Verification items for the finished model (mm, model axes). Face numbers are marked on the shaded views. A direction names the side the tool comes from. Give positions to 0.01 mm unless a question says otherwise; leave off trailing zeros. Write each loop counter-clockwise with the first axis right and the second up, starting at its lowest first coordinate (ties: lowest second). Pieces come first, ordered by that corner, then holes. Notation, with made-up numbers: (85.5, 9) -> (126.5, 9) arc R26 cw to (126.5, 35) -> close; hole circle Ø3 at (12, -29.75). An arc over 180 degrees is marked (long way). Answer as CSV lines item,"result". Start each with the question number.
1) Sectioned sample at A-A on y = 0. Record the cut outline in (x, z), and give its area (3 significant figures).
2) Sectioned sample at C-C on z = 18.5. Record the cut outline in (x, y), and give its area (3 significant figures).
3) Material ranges on L1, parallel to Y at x = 0, z = 5.3; L2, parallel to Y at x = 0, z = 1.45; L3, parallel to X at y = -5, z = 5.5, recorded low to high.
4) Sectioned sample at D-D on z = 1.75. Record the cut outline in (x, y), and give its area (3 significant figures).
5) Mould release check, pull along Y, two halves, no side actions. Record for the marked faces 4, 5 and 6: released by +Y, released by -Y, zero draft, split by the parting line, or undercut.
6) Tool access check on the marked faces 1, 2 and 3. Record the directions out of +Z, -Z, +X, -X, +Y, -Y that give a thin tool (end or side, any length) a straight path to the whole face; none if there is none.
7) Sectioned sample at B-B on x = 0. Record the cut outline in (y, z).
8) Gauge pin test, flat ends, axial feed: pin 1 Ø3 at (y, z) = (7, 3.5) entering from +X; pin 2 Ø1 at (x, z) = (-1, 15) entering from -Y; pin 3 Ø7.5 at (x, y) = (0, 0) entering from -Z; pin 4 Ø1 at (x, y) = (-5, 4) entering from +Z. Record the tip position at first contact, or that the pin passes through.
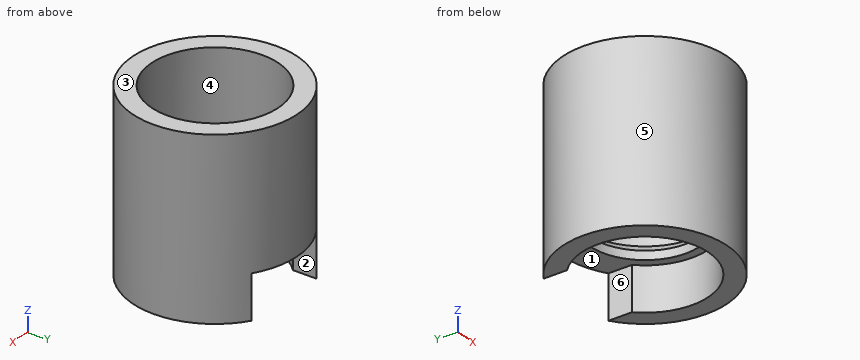
```python
from build123d import *

# Parameters (mm, degrees)
F3_DEPTH = 25


with BuildPart() as f1:
    # F0 (on Front) → F1 (revolve)
    with BuildSketch(Plane.XZ):
        Polygon((7.25, 0), (9.4, 0), (9.4, 20), (7.25, 20), (7.25, 7), (6.25, 6), (6.25, 5), (7.25, 5), align=None)
    revolve(axis=Axis((0, 0, 5), (0, 0, 1)))

    # F2 (on Front) → F3 (cut)
    with BuildSketch(Plane.XZ):
        Polygon((5, 5), (-5, 5), (-5, 0), (0, 0), (5, 0), align=None)
    extrude(amount=-F3_DEPTH, mode=Mode.SUBTRACT)


solid = f1.part
```
Ans:
1,outline,"(-9.4, 0) -> (-7.25, 0) -> (-7.25, 5) -> (-6.25, 5) -> (-6.25, 6) -> (-7.25, 7) -> (-7.25, 20) -> (-9.4, 20) -> close; (6.25, 5) -> (7.25, 5) -> (7.25, 0) -> (9.4, 0) -> (9.4, 20) -> (7.25, 20) -> (7.25, 7) -> (6.25, 6) -> close"
1,area,"89.0 mm²"
2,outline,"circle Ø18.8 at (0, 0); hole circle Ø14.5 at (0, 0)"
2,area,"112 mm²"
3,L1,"y = -9.4 to -6.25, 6.25 to 9.4"
3,L2,"y = -9.4 to -7.25"
3,L3,"x = -7.96 to -3.75, 3.75 to 7.96"
4,outline,"(-5, 5.25) -> (-5, 7.96) arc R9.4 ccw (long way) to (5, 7.96) -> (5, 5.25) arc R7.25 cw (long way) to start"
4,area,"89.4 mm²"
5,face 4,"undercut"
5,face 5,"split by the parting line"
5,face 6,"zero draft"
6,face 1,"-Z"
6,face 2,"-Z, +Y"
6,face 3,"+Z, +X, -X, +Y, -Y"
7,outline,"(-9.4, 0) -> (-7.25, 0) -> (-7.25, 5) -> (-6.25, 5) -> (-6.25, 6) -> (-7.25, 7) -> (-7.25, 20) -> (-9.4, 20) -> close; (6.25, 5) -> (9.4, 5) -> (9.4, 20) -> (7.25, 20) -> (7.25, 7) -> (6.25, 6) -> close"
8,pin 1,"stops at x = 7.62"
8,pin 2,"stops at y = -9.39"
8,pin 3,"passes through"
8,pin 4,"stops at z = 6.65"
